```python
from build123d import *

# Parameters (mm, degrees)
ESQUISSE1_W             = 45
ESQUISSE1_H             = 10
BOSS_EXTRU_1_DEPTH      = 3
ESQUISSE2_R             = 1.625
ENL_V_MAT_EXTRU_1_DEPTH = 4
ESQUISSE3_W             = 5
ESQUISSE3_H             = 3
BOSS_EXTRU_2_DEPTH      = 10
BOSS_EXTRU_2_DEPTH_BACK = 20
ESQUISSE4_W             = 5
ESQUISSE4_H             = 30
BOSS_EXTRU_3_DEPTH      = 10.5
ENL_V_MAT_EXTRU_2_DEPTH = 31


with BuildPart() as part:
    # Esquisse1 → Boss.-Extru.1 (new body)
    with BuildSketch(Plane.XY):
        with Locations((17.5, -5)):
            Rectangle(ESQUISSE1_W, ESQUISSE1_H)
    extrude(amount=BOSS_EXTRU_1_DEPTH)

    # Esquisse2 → Enlèv. mat.-Extru.1 (cut, through all)
    with BuildSketch(Plane.XY.offset(3)):
        with Locations((30, -5)):
            Circle(ESQUISSE2_R)
        with Locations((5, -5)):
            Circle(ESQUISSE2_R)
    extrude(amount=-ENL_V_MAT_EXTRU_1_DEPTH, mode=Mode.SUBTRACT)

    # Esquisse3 → Boss.-Extru.2 (add, two sides)
    with BuildSketch(Plane.XZ.offset(10)) as boss_extru_2_sk:
        with Locations((37.5, 1.5)):
            Rectangle(ESQUISSE3_W, ESQUISSE3_H)
    extrude(amount=BOSS_EXTRU_2_DEPTH)
    extrude(boss_extru_2_sk.sketch, amount=-BOSS_EXTRU_2_DEPTH_BACK)

    # Esquisse4 → Boss.-Extru.3 (add)
    with BuildSketch(Plane.XY.offset(3)):
        with Locations((37.5, -5)):
            Rectangle(ESQUISSE4_W, ESQUISSE4_H)
    extrude(amount=BOSS_EXTRU_3_DEPTH)

    # Esquisse5 → Enlèv. mat.-Extru.2 (cut, through all)
    with BuildSketch(Plane.XZ.offset(20)):
        Polygon((35, 13.5), (40, 13.5), (35, 13.4), align=None)
    extrude(amount=-ENL_V_MAT_EXTRU_2_DEPTH, mode=Mode.SUBTRACT)


solid = part.part
```
CAD build for the part. Positions are in the model's coordinates, mm. A direction names the side the tool comes from. Give positions to 0.01 mm unless a question says otherwise; leave off trailing zeros. Order: outer loops, then holes, each group sorted by start corner. A loop starts at its lowest first (then second) coordinate and runs counter-clockwise, first axis right, second up.
(1) Saw through at D-D, the plane y = 6. Give the cut face in (x, z), then the cut area to 4 significant figures.
(2) Saw through at B-B, the plane y = -5. Give the cut face in (x, z) (3 decimals), then the cut area to 3 significant figures.
(3) Saw through at C-C, the plane z = 1. Give the cut face in (x, y) (3 decimals), then the cut area to 3 significant figures.
(4) Saw through at A-A, the plane x = 30. Give the cut face in (y, z) (3 decimals).
(5) Mould opens along Y. For faces 6 (the flat face through (37, 10, 7)), 7 (the flat face through (40, -5, 7)), 8 (the cylindrical face through (3.802, -3.902, 1.521)) say: released by +Y, released by -Y, zero draft, split by the parting line, or undercut.
(6) Tool access for faces 1 (the flat face through (-5, -5, 1)), 2 (the flat face through (15, -5, 3)), 3 (the flat face through (22, -5, 0)), 4 (the flat face through (15, -10, 1)), 5 (the flat face through (15, 0, 1)): list every direction of +Z, -Z, +X, -X, +Y, -Y with a clear straight run to the whole face (end or side of a thin tool).
(7) Flat gauge pins, fed straight in: pin 1 (2.5 mm diameter, centred on x = 11.5, z = 1.5, fed in from -Y); pin 2 (1.5 mm diameter, centred on x = 13, y = -1, fed in from -Z); pin 3 (2 mm diameter, centred on x = 32.5, y = -3.5, fed in from +Z); pin 4 (3.5 mm diameter, centred on x = 18, z = 2, fed in from +Y). Where does each tip first touch, or does it go through?
(8) Drill centre lines: L1, parallel to Y at x = 5, z = 1.75 (3 decimals); L2, parallel to X at y = -11, z = 8.5; L3, parallel to Y at x = 19.5, z = 1.5. Where is each one in solid material? Low to high.
Results found:
1. outline: (35, 0) - (40, 0) - (40, 13.5) - (35, 13.4) - close
1. area: 67.25 mm2
2. outline: (-5, 0) - (3.375, 0) - (3.375, 3) - (-5, 3) - close; (6.625, 0) - (28.375, 0) - (28.375, 3) - (6.625, 3) - close; (31.625, 0) - (40, 0) - (40, 13.5) - (35, 13.4) - (35, 3) - (31.625, 3) - close
2. area: 168 mm2
3. outline: (-5, -10) - (35, -10) - (35, -20) - (40, -20) - (40, 10) - (35, 10) - (35, 0) - (-5, 0) - close; hole circle Ø3.25 at (5, -5); hole circle Ø3.25 at (30, -5)
3. area: 533 mm2
4. outline: (-10, 0) - (-6.625, 0) - (-6.625, 3) - (-10, 3) - close; (-3.375, 0) - (0, 0) - (0, 3) - (-3.375, 3) - close
5. face 6: released by +Y
5. face 7: zero draft
5. face 8: undercut
6. face 1: +Z, -Z, -X, +Y, -Y
6. face 2: +Z, -X, +Y, -Y
6. face 3: -Z, +X, -X, +Y, -Y
6. face 4: +Z, -Z, -X, -Y
6. face 5: +Z, -Z, -X, +Y
7. pin 1: stops at y = -10
7. pin 2: stops at z = 0
7. pin 3: stops at z = 3
7. pin 4: stops at y = 0
8. L1: y = -10 to -6.625, -3.375 to 0
8. L2: x = 35 to 40
8. L3: y = -10 to 0
